Could you check a few things on this model? Use its own coordinates, in mm. A direction names the side the tool comes from. Give positions to 0.01 mm unless a question says otherwise; leave off trailing zeros. Order: outer loops, then holes, each group sorted by start corner. A loop starts at its lowest first (then second) coordinate and runs counter-clockwise, first axis right, second up. Notation, with made-up numbers: M 54,2 L 82,2 A26 cw 82,27 Z; hole C -5.75,54 d5. An arc over 180 degrees is marked long. Use a Markdown table: item, result. Add a question column.
Item 1: If I drill on L1, parallel to Z at x = 34.5, y = 19; L2, parallel to Z at x = 10.5, y = 38; L3, parallel to Y at x = 20, z = -51, over which ranges is the centre line in solid material (lowest first)? Write a range as from..to.
Item 2: I'm going to push flat-ended pins straight in: pin 1 Ø1.9 at (x, z) = (-3, 4.5) entering from +Y; pin 2 Ø4 at (x, z) = (-19.5, -61) entering from -Y; pin 3 Ø1.5 at (x, z) = (-22.5, -18.5) entering from +Y (3 decimals). Where does each tip first touch, or does it pass through?
Item 3: Suppose I cut it at C-C on z = -20. Write out the boundary of the cut face in (x, y) (3 decimals), plus the area to 3 significant figures.
Item 4: If we mould it in two halves opening along Z, with no side actions, what happens to faces 1 (the face through (-35.66, 20.19, -109.56)), 2 (the face through (35.66, 20.19, 4.74)), 3 (the face through (0, 31.75, 3)), 4 (the face through (22.22, 38.99, -53.22))? For each: released by +Z, released by -Z, zero draft, split by the parting line, or undercut.
Item 5: Suppose I cut it at A-A on x = 13. Write out the boundary of the cut face in (y, z) (3 decimals), plus the area to 3 significant figures.
Item 6: Suppose I cut it at B-B on y = -14. Write out the boundary of the cut face in (x, z) (3 decimals).
Item 7: For faces 5 (the face through (-35.623, -20.17, 1.565)), 6 (the face through (35.28, 20.77, -109.52)), 7 (the face through (27.368, -16.097, -111.081)), which set-ups out of +Z, -Z, +X, -X, +Y, -Y let a thin tool reach every point of the face, with its end or its side?
from build123d import *

# Parameters (mm, degrees)
F1_DEPTH     = 6.35
F2_T1_DEPTH  = 77.4547380887
F3_T1_DEPTH  = 71.5888593537
F4_T1_DEPTH  = 71.5888593537
F5_T1_DEPTH  = 71.5888593537
F6_T1_DEPTH  = 71.5888593537
F7_T1_DEPTH  = 65.7229806188
F11_DEPTH    = 6.35
F12_T1_DEPTH = 77.4547380887
F13_T1_DEPTH = 71.5888593537
F14_T1_DEPTH = 71.5888593537
F15_T1_DEPTH = 71.5888593537
F16_T1_DEPTH = 71.5888593537
F17_T1_DEPTH = 65.7229806188
F18_DEPTH    = 107.95


# Not quite as in the source:
# - a fillet or chamfer that OpenCascade refuses, or shapes differently, is made with other operations: its cross-section is extruded or revolved along the edge and cut away or added


with BuildPart() as f1:
    # F0 (on Top) → F1 (new body)
    with BuildSketch(Plane.XY):
        Polygon((25.6632194655, 44.45), (-25.6632194655, 44.45), (-51.326438931, 0), (-25.6632194655, -44.45), (25.6632194655, -44.45), (51.326438931, 0), align=None)
        Polygon((-36.6617420935, 0), (-18.3308710468, 31.75), (18.3308710468, 31.75), (36.6617420935, 0), (18.3308710468, -31.75), (-18.3308710468, -31.75), align=None, mode=Mode.SUBTRACT)
    extrude(amount=F1_DEPTH)

    # F2: chamfer of 5.08 on 2 edges, made by hand

    # F2_s2 → F2_t1 (cut)
    with BuildSketch(Plane.YZ.offset(-38.7273690443)):
        Polygon((-44.45, 5.08), (-39.37, 0), (-44.45, 0), align=None)
        Polygon((-44.45, 1.27), (-39.37, 6.35), (-44.45, 6.35), align=None)
    extrude(amount=F2_T1_DEPTH, mode=Mode.SUBTRACT)

    # F3: chamfer of 5.08 on 2 edges, made by hand

    # F3_s2 → F3_t1 (cut)
    with BuildSketch(Plane(origin=(-16.4307451547, -28.4588854141, 0), x_dir=(0, 0, 1), z_dir=(0.5, 0.8660254038, 0))):
        Polygon((0, 39.37), (5.08, 44.45), (0, 44.45), align=None)
        Polygon((6.35, 39.37), (1.27, 44.45), (6.35, 44.45), align=None)
    extrude(amount=F3_T1_DEPTH, mode=Mode.SUBTRACT)

    # F4: chamfer of 5.08 on 2 edges, made by hand

    # F4_s2 → F4_t1 (cut)
    with BuildSketch(Plane(origin=(16.4307451547, -28.4588854141, 0), x_dir=(0, 0, 1), z_dir=(-0.5, 0.8660254038, 0))):
        Polygon((5.08, 44.45), (0, 39.37), (0, 44.45), align=None)
        Polygon((1.27, 44.45), (6.35, 39.37), (6.35, 44.45), align=None)
    extrude(amount=F4_T1_DEPTH, mode=Mode.SUBTRACT)

    # F5: chamfer of 5.08 on 2 edges, made by hand

    # F5_s2 → F5_t1 (cut)
    with BuildSketch(Plane.YZ.offset(-38.7273690443)):
        Polygon((44.45, 5.08), (39.37, 0), (44.45, 0), align=None)
        Polygon((44.45, 1.27), (39.37, 6.35), (44.45, 6.35), align=None)
    extrude(amount=F5_T1_DEPTH, mode=Mode.SUBTRACT)

    # F6: chamfer of 5.08 on 2 edges, made by hand

    # F6_s2 → F6_t1 (cut)
    with BuildSketch(Plane(origin=(16.4307451547, 28.4588854141, 0), x_dir=(0, 0, 1), z_dir=(-0.5, -0.8660254038, 0))):
        Polygon((0, 39.37), (5.08, 44.45), (0, 44.45), align=None)
        Polygon((1.27, 44.45), (6.35, 39.37), (6.35, 44.45), align=None)
    extrude(amount=F6_T1_DEPTH, mode=Mode.SUBTRACT)

    # F7: chamfer of 5.08 on 2 edges, made by hand

    # F7_s2 → F7_t1 (cut)
    with BuildSketch(Plane(origin=(-16.4307451547, 28.4588854141, 0), x_dir=(0, 0, 1), z_dir=(0.5, -0.8660254038, 0))):
        Polygon((0, 39.37), (5.08, 44.45), (0, 44.45), align=None)
        Polygon((1.27, 44.45), (6.35, 39.37), (6.35, 44.45), align=None)
    extrude(amount=F7_T1_DEPTH, mode=Mode.SUBTRACT)



with BuildPart() as f11:
    # F10 (on offset) → F11 (new body)
    with BuildSketch(Plane(origin=(0, 0, -107.95), x_dir=(1, 0, 0), z_dir=(0, 0, -1))):
        Polygon((25.6632194655, 44.45), (-25.6632194655, 44.45), (-51.326438931, 0), (-25.6632194655, -44.45), (25.6632194655, -44.45), (51.326438931, 0), align=None)
        Polygon((-36.6617420935, 0), (-18.3308710468, 31.75), (18.3308710468, 31.75), (36.6617420935, 0), (18.3308710468, -31.75), (-18.3308710468, -31.75), align=None, mode=Mode.SUBTRACT)
    extrude(amount=F11_DEPTH)

    # F12: chamfer of 5.08 on 2 edges, made by hand

    # F12_s2 → F12_t1 (cut)
    with BuildSketch(Plane(origin=(-19.3636845222, -33.5388854141, 0), x_dir=(0, 0, 1), z_dir=(0.5, 0.8660254038, 0))):
        Polygon((-109.22, -44.45), (-114.3, -39.37), (-114.3, -44.45), align=None)
        Polygon((-113.03, -44.45), (-107.95, -39.37), (-107.95, -44.45), align=None)
    extrude(amount=F12_T1_DEPTH, mode=Mode.SUBTRACT)

    # F13: chamfer of 5.08 on 2 edges, made by hand

    # F13_s2 → F13_t1 (cut)
    with BuildSketch(Plane(origin=(19.3636845222, -33.5388854141, 0), x_dir=(0, 0, 1), z_dir=(-0.5, 0.8660254038, 0))):
        Polygon((-109.22, -44.45), (-114.3, -39.37), (-114.3, -44.45), align=None)
        Polygon((-113.03, -44.45), (-107.95, -39.37), (-107.95, -44.45), align=None)
    extrude(amount=F13_T1_DEPTH, mode=Mode.SUBTRACT)

    # F14: chamfer of 5.08 on 2 edges, made by hand

    # F14_s2 → F14_t1 (cut)
    with BuildSketch(Plane.YZ.offset(-32.8614903094)):
        Polygon((-44.45, -113.03), (-39.37, -107.95), (-44.45, -107.95), align=None)
        Polygon((-44.45, -109.22), (-39.37, -114.3), (-44.45, -114.3), align=None)
    extrude(amount=F14_T1_DEPTH, mode=Mode.SUBTRACT)

    # F15: chamfer of 5.08 on 2 edges, made by hand

    # F15_s2 → F15_t1 (cut)
    with BuildSketch(Plane(origin=(19.3636845222, 33.5388854141, 0), x_dir=(0, 0, 1), z_dir=(-0.5, -0.8660254038, 0))):
        Polygon((-107.95, -39.37), (-113.03, -44.45), (-107.95, -44.45), align=None)
        Polygon((-109.22, -44.45), (-114.3, -39.37), (-114.3, -44.45), align=None)
    extrude(amount=F15_T1_DEPTH, mode=Mode.SUBTRACT)

    # F16: chamfer of 5.08 on 2 edges, made by hand

    # F16_s2 → F16_t1 (cut)
    with BuildSketch(Plane(origin=(-19.3636845222, 33.5388854141, 0), x_dir=(0, 0, 1), z_dir=(0.5, -0.8660254038, 0))):
        Polygon((-107.95, -39.37), (-113.03, -44.45), (-107.95, -44.45), align=None)
        Polygon((-109.22, -44.45), (-114.3, -39.37), (-114.3, -44.45), align=None)
    extrude(amount=F16_T1_DEPTH, mode=Mode.SUBTRACT)

    # F17: chamfer of 5.08 on 2 edges, made by hand

    # F17_s2 → F17_t1 (cut)
    with BuildSketch(Plane.YZ.offset(-32.8614903094)):
        Polygon((39.37, -107.95), (44.45, -113.03), (44.45, -107.95), align=None)
        Polygon((44.45, -109.22), (39.37, -114.3), (44.45, -114.3), align=None)
    extrude(amount=F17_T1_DEPTH, mode=Mode.SUBTRACT)


with BuildPart() as f1_1:
    add(f1.part)

    add(f11.part)  # F18 merges F11
    # F8 (on face) → F18 (join)
    with BuildSketch(Plane(origin=(0, 0, 0), x_dir=(1, 0, 0), z_dir=(0, 0, -1))):
        with BuildLine():
            ThreePointArc((-24.4019218999, 36.4746314671), (-22.996261449, 32.0179739378), (-18.3308710468, 31.75))
            ThreePointArc((-18.3308710468, 31.75), (-16.8828037041, 33.2488412093), (-16.3549710973, 35.2649802766))
            ThreePointArc((-16.3549710973, 35.2649802766), (-17.4635050287, 38.0744368309), (-20.1917663217, 39.37))
            Line((-20.1917663217, 39.37), (-20.7469664852, 39.37))
            ThreePointArc((-20.7469664852, 39.37), (-22.2395757858, 38.9790895208), (-23.4832328124, 38.065847643))
            Line((-23.4832328124, 38.065847643), (-24.4019218999, 36.4746314671))
        make_face()
        with BuildLine():
            ThreePointArc((-44.2711808809, -2.0600654032), (-39.7103407865, -3.8229800416), (-36.6617420935, 0))
            ThreePointArc((-36.6617420935, 0), (-36.6592700651, 0.0824842573), (-36.6584459461, 0.165001434))
            ThreePointArc((-36.6584459461, 0.165001434), (-39.1605946831, 3.9616727057), (-43.6363324768, 3.1596550942))
            Line((-43.6363324768, 3.1596550942), (-44.8066059423, 1.1326819932))
            ThreePointArc((-44.8066059423, 1.1326819932), (-44.8913049977, -0.3338212735), (-44.4575484053, -1.7372673821))
            Line((-44.4575484053, -1.7372673821), (-44.2711808809, -2.0600654032))
        make_face()
        with BuildLine():
            ThreePointArc((20.1917663217, 39.37), (16.4724326672, 36.2410793716), (18.3308710468, 31.75))
            ThreePointArc((18.3308710468, 31.75), (22.4855054708, 31.6784175772), (24.5837617096, 35.2649802766))
            ThreePointArc((24.5837617096, 35.2649802766), (24.5380477999, 35.8766014255), (24.4019218999, 36.4746314671))
            Line((24.4019218999, 36.4746314671), (23.4832328124, 38.065847643))
            ThreePointArc((23.4832328124, 38.065847643), (22.2395757858, 38.9790895208), (20.7469664852, 39.37))
            Line((20.7469664852, 39.37), (20.1917663217, 39.37))
        make_face()
        with BuildLine():
            ThreePointArc((43.6363324768, 3.1596550942), (39.0850907082, 3.9283723543), (36.6617420935, 0))
            ThreePointArc((36.6617420935, 0), (39.7103407865, -3.8229800416), (44.2711808809, -2.0600654032))
            Line((44.2711808809, -2.0600654032), (44.4575484053, -1.7372673821))
            ThreePointArc((44.4575484053, -1.7372673821), (44.8038576253, -0.8140164387), (44.9215282886, 0.165001434))
            ThreePointArc((44.9215282886, 0.165001434), (44.8926971055, 0.6522418291), (44.8066059423, 1.1326819932))
            Line((44.8066059423, 1.1326819932), (43.6363324768, 3.1596550942))
        make_face()
        with BuildLine():
            ThreePointArc((24.5837617096, -35.2649802766), (22.4855054708, -31.6784175772), (18.3308710468, -31.75))
            ThreePointArc((18.3308710468, -31.75), (16.4724326672, -36.2410793716), (20.1917663217, -39.37))
            Line((20.1917663217, -39.37), (20.7469664852, -39.37))
            ThreePointArc((20.7469664852, -39.37), (22.2395757858, -38.9790895208), (23.4832328124, -38.065847643))
            Line((23.4832328124, -38.065847643), (24.4019218999, -36.4746314671))
            ThreePointArc((24.4019218999, -36.4746314671), (24.5380477999, -35.8766014255), (24.5837617096, -35.2649802766))
        make_face()
        with BuildLine():
            ThreePointArc((-16.3549710973, -35.2649802766), (-16.8828037041, -33.2488412093), (-18.3308710468, -31.75))
            ThreePointArc((-18.3308710468, -31.75), (-22.996261449, -32.0179739378), (-24.4019218999, -36.4746314671))
            Line((-24.4019218999, -36.4746314671), (-23.4832328124, -38.065847643))
            ThreePointArc((-23.4832328124, -38.065847643), (-22.2395757858, -38.9790895208), (-20.7469664852, -39.37))
            Line((-20.7469664852, -39.37), (-20.1917663217, -39.37))
            ThreePointArc((-20.1917663217, -39.37), (-17.4635050287, -38.0744368309), (-16.3549710973, -35.2649802766))
        make_face()
    extrude(amount=F18_DEPTH)


solid = f1_1.part
Findings below:
| question | item | result |
|---|---|---|
| 1 | L1 | z = -114.29..-107.96, 0.01..6.34 |
| 1 | L2 | z = -114.3..-107.95, 0..6.35 |
| 1 | L3 | y = -39.35..-31.18, 31.18..39.35 |
| 2 | pin 1 | stops at y = 42.17 |
| 2 | pin 2 | stops at y = -39.37 |
| 2 | pin 3 | stops at y = 39.175 |
| 3 | outline | M -44.807,-1.133 L -43.636,-3.16 A4.132 ccw long -44.271,2.06 L -44.458,1.737 A4.132 ccw Z; M -24.402,-36.475 L -23.483,-38.066 A4.114 ccw -20.747,-39.37 L -20.192,-39.37 A4.114 ccw long Z; M -24.402,36.475 A4.114 ccw long -20.192,39.37 L -20.747,39.37 A4.114 ccw -23.483,38.066 Z; M 20.192,-39.37 L 20.747,-39.37 A4.114 ccw 23.483,-38.066 L 24.402,-36.475 A4.114 ccw long Z; M 20.192,39.37 A4.114 ccw long 24.402,36.475 L 23.483,38.066 A4.114 ccw 20.747,39.37 Z; M 43.636,-3.16 L 44.807,-1.133 A4.132 ccw 44.458,1.737 L 44.271,2.06 A4.132 ccw long Z |
| 3 | area | 319 mm^2 |
| 4 | face 1 | undercut |
| 4 | face 2 | released by +Z |
| 4 | face 3 | zero draft |
| 4 | face 4 | undercut |
| 5 | outline | M -42.545,-111.125 L -39.37,-114.3 L -31.75,-114.3 L -31.75,-107.95 L -39.37,-107.95 Z; M -42.545,3.175 L -39.37,0 L -31.75,0 L -31.75,6.35 L -39.37,6.35 Z; M 31.75,-114.3 L 39.37,-114.3 L 42.545,-111.125 L 39.37,-107.95 L 31.75,-107.95 Z; M 31.75,0 L 39.37,0 L 42.545,3.175 L 39.37,6.35 L 31.75,6.35 Z |
| 5 | area | 234 mm^2 |
| 6 | outline | M -41.044,-111.125 L -37.378,-114.3 L -28.579,-114.3 L -28.579,-107.95 L -37.378,-107.95 Z; M -41.044,3.175 L -37.378,0 L -28.579,0 L -28.579,6.35 L -37.378,6.35 Z; M 28.579,-114.3 L 37.378,-114.3 L 41.044,-111.125 L 37.378,-107.95 L 28.579,-107.95 Z; M 28.579,0 L 37.378,0 L 41.044,3.175 L 37.378,6.35 L 28.579,6.35 Z |
| 7 | face 5 | -X, -Y |
| 7 | face 6 | +X, +Y |
| 7 | face 7 | +Z, -Z |
